The figure shows three views and two pictorial views of one solid part (mm, origin at its lowest corner). Answer the questions. Coordinates: 2 decimals unless noted, no trailing zeros. Write each loop counter-clockwise with the first axis right and the second up, starting at its lowest first coordinate (ties: lowest second). Pieces come first, ordered by that corner, then holes.
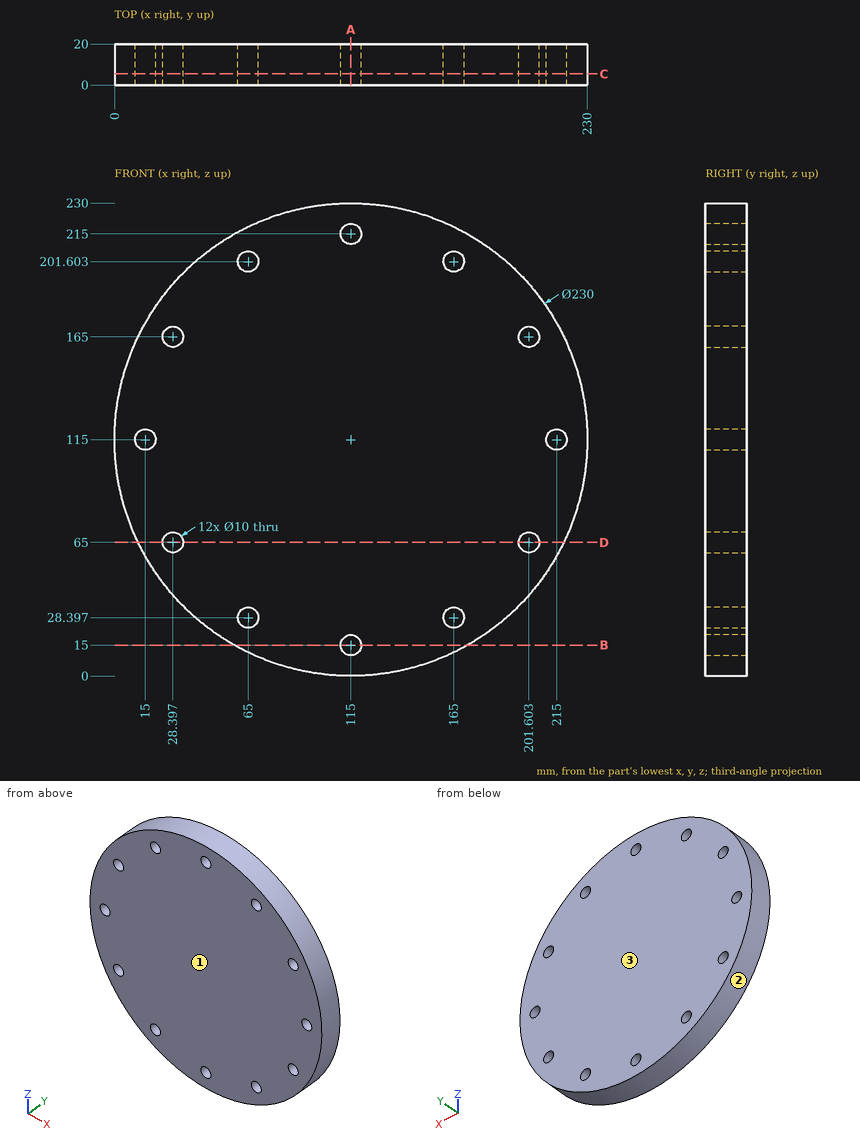
Item 1: The part is cut by section A-A (x = 115). Give the vertices of the cut face in (y, z).
Item 2: Given pin 1 (5 mm diameter, centred on y = 10, z = 44.5, fed in from -X); pin 2 (3 mm diameter, centred on y = 7.5, z = 135.5, fed in from +X); pin 3 (10 mm diameter, centred on y = 14, z = 181.5, fed in from -X) (1 decimal), each flat-ended and moving along its own axis, determine where each tip first touches the part or whether it passes through.
Item 3: The part is cut by section D-D (z = 65). Give the vertices of the cut face in (x, y).
Item 4: The part is cut by section B-B (z = 15). Give the vertices of the cut face in (x, y), and give its area (3 significant figures).
Item 5: Find the intervals of material crossed by probe 1 along Z at (x, y) = (161, 11) (1 decimal); probe 2 along X at (y, z) = (4.5, 115); probe 3 along Z at (x, y) = (206, 6.25) (1 decimal), in increasing order.
Item 6: The part is cut by section C-C (y = 5.5). State how many separate pieces and enclosed holes the cut face has, and give its area (3 significant figures).
Item 7: Determine the mould class of the marked faces 1, 2 and 3 for opening direction Y: +Y half, -Y half, draft (parallel to the pull), parting line (faces both ways), or undercut.
Answer:
1. outline: (0, 0) - (20, 0) - (20, 10) - (0, 10) - close; (0, 20) - (20, 20) - (20, 210) - (0, 210) - close; (0, 220) - (20, 220) - (20, 230) - (0, 230) - close
2. pin 1: stops at x = 22.26
2. pin 2: stops at x = 228.42
2. pin 3: stops at x = 17.8
3. outline: (11.44, 0) - (23.4, 0) - (23.4, 20) - (11.44, 20) - close; (33.4, 0) - (196.6, 0) - (196.6, 20) - (33.4, 20) - close; (206.6, 0) - (218.56, 0) - (218.56, 20) - (206.6, 20) - close
4. outline: (58.21, 0) - (110, 0) - (110, 20) - (58.21, 20) - close; (120, 0) - (171.79, 0) - (171.79, 20) - (120, 20) - close
4. area: 2,070 mm2
5. probe 1: z = 9.6 to 25.4, 31.4 to 198.6, 204.6 to 220.4
5. probe 2: x = 0 to 10, 20 to 210, 220 to 230
5. probe 3: z = 44.7 to 62.6, 67.4 to 162.6, 167.4 to 185.3
6. separate pieces: 1
6. enclosed holes: 12
6. area: 40,600 mm2
7. face 1: -Y half
7. face 2: draft
7. face 3: +Y half
